Build history of the part. All positions in model axes, mm. Coordinates: 2 decimals unless noted, no trailing zeros.
from build123d import *

# Parameters (mm, degrees)
CROQUIS1_W              = 84.5
CROQUIS1_H              = 62
CROQUIS1_R              = 1.65
SALIENTE_EXTRUIR1_DEPTH = 22
REDONDEO1_R             = 3


with BuildPart() as part:
    # Croquis1 → Saliente-Extruir1 (new body)
    with BuildSketch(Plane.XY):
        with Locations((42.25, 31)):
            Rectangle(CROQUIS1_W, CROQUIS1_H)
        with Locations((3, 3)):
            Circle(CROQUIS1_R, mode=Mode.SUBTRACT)
        with Locations((81.5, 3)):
            Circle(CROQUIS1_R, mode=Mode.SUBTRACT)
        with Locations((81.5, 59)):
            Circle(CROQUIS1_R, mode=Mode.SUBTRACT)
        with Locations((3, 59)):
            Circle(CROQUIS1_R, mode=Mode.SUBTRACT)
    extrude(amount=SALIENTE_EXTRUIR1_DEPTH)

    # Redondeo1
    redondeo1_edges = [part.edges().sort_by_distance(p)[0] for p in [
        (0, 62, 11),
        (84.5, 62, 11),
        (84.5, 0, 11),
        (0, 0, 11),
    ]]
    fillet(redondeo1_edges, radius=REDONDEO1_R)


solid = part.part
(1) Flat gauge pin, fed straight in: P1, Ø3, axis at x = 81.5, y = 3, coming from the -Z side. Where does the tip first touch, or does it go through?
(2) Two-plate mould, pull along Y, no slides. Class faces 1 (the flat face through (42, 31, 0)), 2 (the cylindrical face through (2.6, 57.4, 10.8)), 3 (the cylindrical face through (83.6, 61.14, 11.15)), 4 (the flat face through (42, 0, 11)): pulls with the +Y half, pulls with the -Y half, needs draft (parallel to the pull), parting line crosses it, or undercut.
(3) Probe L1, parallel to Y at x = 3, z = 17; L2, parallel to Y at x = 80.5, z = 6.75. List the from-to ranges inside material, lowest first.
Results:
1. P1: passes through
2. face 1: needs draft
2. face 2: undercut
2. face 3: pulls with the +Y half
2. face 4: pulls with the -Y half
3. L1: y = 0 to 1.35, 4.65 to 57.35, 60.65 to 62
3. L2: y = 0 to 1.69, 4.31 to 57.69, 60.31 to 62
